Input: part model. Units: mm. Frame: model coordinates. Give positions to 0.01 mm unless a question says otherwise; leave off trailing zeros. Order: outer loops, then holes, each group sorted by start corner. A loop starts at its lowest first (then second) coordinate and runs counter-clockwise, first axis right, second up. Notation, with made-up numbers: M -33,68 L 19,68 A19 cw 19,94 Z; hole C -9.75,12.5 d5. An arc over 180 degrees is marked long. Use a Markdown table: item, result.
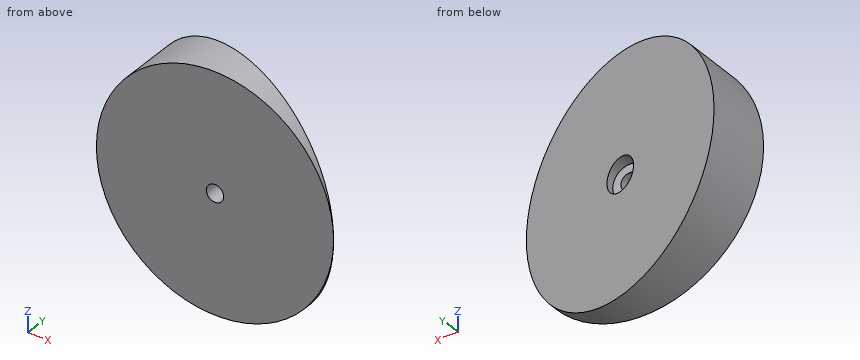
from build123d import *

# Parameters (mm, degrees)
SKETCH1_R               = 55
SKETCH1_R_2             = 4
BOSS_EXTRUDE1_DEPTH     = 32
CUT_EXTRUDE1_DEPTH      = 56
CUT_EXTRUDE1_DEPTH_BACK = 56
SKETCH4_R               = 7.796617101
CUT_EXTRUDE2_DEPTH      = 23


with BuildPart() as part:
    # Sketch1 → Boss-Extrude1 (new body)
    with BuildSketch(Plane(origin=(0, 0, 0), x_dir=(1, 0, 0), z_dir=(0, 1, 0))):
        Circle(SKETCH1_R)
        Circle(SKETCH1_R_2, mode=Mode.SUBTRACT)
    extrude(amount=BOSS_EXTRUDE1_DEPTH)

    # Sketch3 → Cut-Extrude1 (cut, two sides)
    with BuildSketch(Plane.XY) as cut_extrude1_sk:
        Polygon((55, 0), (55, 32), (-55, 32), align=None)
    extrude(amount=CUT_EXTRUDE1_DEPTH, mode=Mode.SUBTRACT)
    extrude(cut_extrude1_sk.sketch, amount=-CUT_EXTRUDE1_DEPTH_BACK, mode=Mode.SUBTRACT)

    # Sketch4 → Cut-Extrude2 (cut, through all)
    with BuildSketch(Plane(origin=(0, 10, 0), x_dir=(1, 0, 0), z_dir=(0, 1, 0))):
        Circle(SKETCH4_R)
    extrude(amount=CUT_EXTRUDE2_DEPTH, mode=Mode.SUBTRACT)


solid = part.part
1) Cut plane C-C on y = 7.5. Return loops of the section in (x, z).
Response values:
| item | result |
|---|---|
| outline | M 29.22,-46.6 L 29.22,46.6 A55 ccw long Z; hole C 0,0 d8 |
2) Cut plane D-D on x = 20. Return loops of the section in (y, z).
Response values:
| item | result |
|---|---|
| outline | M 0,-51.23 L 10.18,-51.23 L 10.18,51.23 L 0,51.23 Z |
3) Cut plane B-B on z = -44.5. Return loops of the section in (x, y), and give its area (3 significant figures).
Response values:
| item | result |
|---|---|
| outline | M -32.32,0 L 32.32,0 L 32.32,6.6 L -32.32,25.4 Z |
| area | 1,030 mm² |
4) First-contact query: pin 1 Ø8 at (x, z) = (3.5, -3.5) entering from +Y; pin 2 Ø5 at (x, z) = (30.5, 6) entering from +Y; pin 3 Ø1 at (y, z) = (17, 1) entering from -X; pin 4 Ø5 at (x, z) = (0, 0) entering from +Y. Flat tips, straight axial feed; report the tip coordinate or a pass-through.
Response values:
| item | result |
|---|---|
| pin 1 | stops at y = 15.27 |
| pin 2 | stops at y = 7.85 |
| pin 3 | stops at x = -55 |
| pin 4 | passes through |
5) Cut plane A-A on x = 0. Return loops of the section in (y, z), and give its area (3 significant figures).
Response values:
| item | result |
|---|---|
| outline | M 0,-55 L 16,-55 L 16,-7.8 L 10,-7.8 L 10,-4 L 0,-4 Z; M 0,4 L 10,4 L 10,7.8 L 16,7.8 L 16,55 L 0,55 Z |
| area | 1,590 mm² |
6) Material intervals for line 1 (Z direction, x = 0, y = 15); line 2 (X direction, y = 14.25, z = 0); line 3 (Z direction, x = -25.5, y = 14), sorted ascending. Write a range as from..to.
Response values:
| item | result |
|---|---|
| line 1 | z = -55..-7.8, 7.8..55 |
| line 2 | x = -55..-7.8 |
| line 3 | z = -48.73..48.73 |
